Input: dimensioned drawing with shaded views. Units: mm. Origin: part minimum x, y, z. A direction names the side the tool comes from. Round coordinates to 2 decimals unless told otherwise and drop trailing zeros. Write each loop counter-clockwise with the first axis right and the second up, starting at its lowest first coordinate (ties: lowest second). Pieces come first, ordered by that corner, then holes. Notation, with made-up numbers: M 81,-35 L 136,-35 A22 cw 136,-3 Z; hole C 53,83 d7. An arc over 180 degrees is marked long. Put each result on its own line as item: value. Start each with the question number.
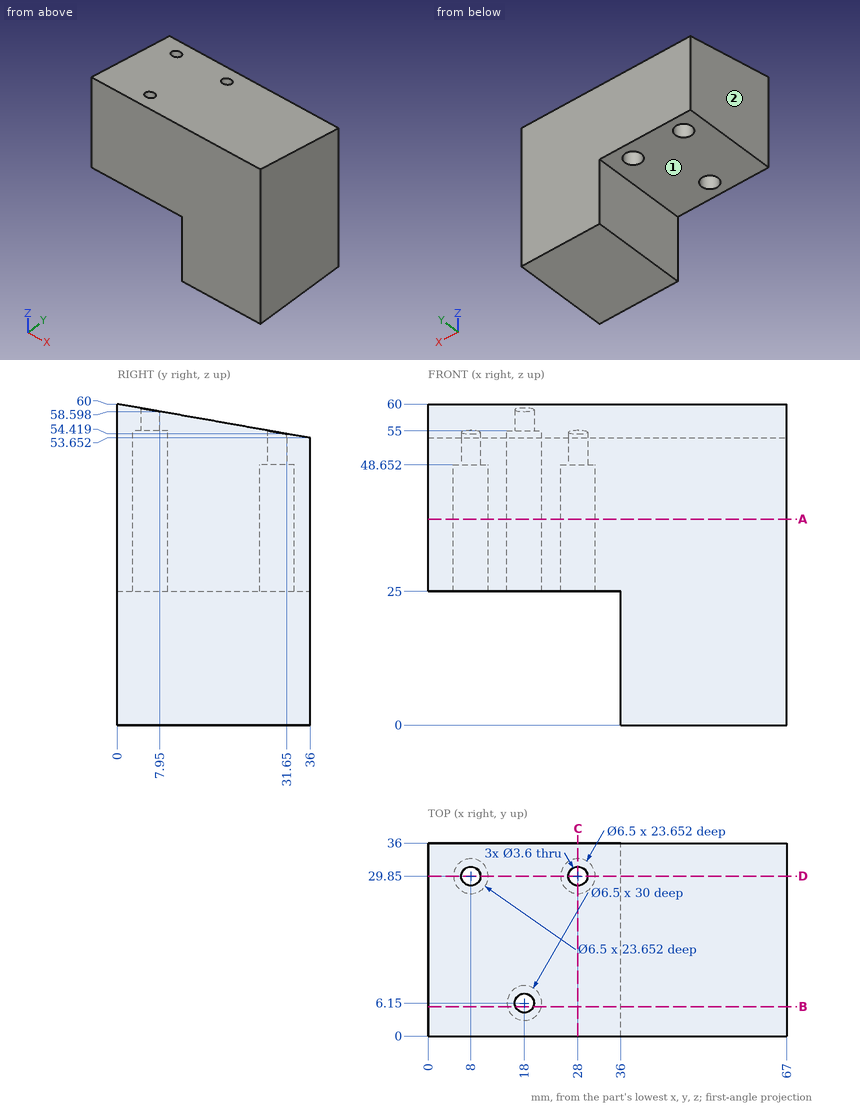
1) Access query for the marked faces 1 and 2. Directions: +Z, -Z, +X, -X, +Y, -Y. A direction counts if a zero-diameter tool reaches every point of the face in a straight line with its end or side. Return the directions, or none.
2) Section C-C, the plane x = 28. Output: boundary loops of the cut face in (y, z).
3) Ray query, probe 1 along X at (y, z) = (29.85, 51.5); probe 2 along X at (y, z) = (29, 35); probe 3 along Y at (x, z) = (18, 31). Return the intervals inside material, ascending.
4) Section A-A, the plane z = 38.5. Output: boundary loops of the cut face in (x, y), and give its area (3 significant figures).
5) First-contact query: pin 1 (7.5 mm diameter, centred on x = 8, y = 29.85, fed in from -Z); pin 2 (6 mm diameter, centred on x = 18, y = 6.15, fed in from +Z); pin 3 (4.5 mm diameter, centred on x = 8, y = 29.85, fed in from -Z); pin 4 (2 mm diameter, centred on x = 8, y = 30.5, fed in from -Z). Flat tips, straight axial feed; report the tip coordinate or a pass-through.
6) Section B-B, the plane y = 5.5. Output: boundary loops of the cut face in (x, z), and give its area (3 significant figures).
7) Section D-D, the plane y = 29.85. Output: boundary loops of the cut face in (x, z), and give its area (3 significant figures).
Solved:
1. face 1: -Z, -X, +Y, -Y
1. face 2: +Z, -Z, -X, +Y, -Y
2. outline: M 0,25 L 26.6,25 L 26.6,48.65 L 28.05,48.65 L 28.05,55.05 L 0,60 Z; M 31.65,48.65 L 33.1,48.65 L 33.1,25 L 36,25 L 36,53.65 L 31.65,54.42 Z
3. probe 1: x = 0 to 6.2, 9.8 to 26.2, 29.8 to 67
3. probe 2: x = 0 to 4.86, 11.14 to 24.86, 31.14 to 67
3. probe 3: y = 0 to 2.9, 9.4 to 36
4. outline: M 0,0 L 67,0 L 67,36 L 0,36 Z; hole C 8,29.85 d6.5; hole C 18,6.15 d6.5; hole C 28,29.85 d6.5
4. area: 2,310 mm2
5. pin 1: stops at z = 25
5. pin 2: stops at z = 59.44
5. pin 3: stops at z = 48.65
5. pin 4: passes through
6. outline: M 0,25 L 14.82,25 L 14.82,55 L 16.32,55 L 16.32,59.03 L 0,59.03 Z; M 19.68,55 L 21.18,55 L 21.18,25 L 36,25 L 36,0 L 67,0 L 67,59.03 L 19.68,59.03 Z
6. area: 2,850 mm2
7. outline: M 0,25 L 4.75,25 L 4.75,48.65 L 6.2,48.65 L 6.2,54.74 L 0,54.74 Z; M 9.8,48.65 L 11.25,48.65 L 11.25,25 L 24.75,25 L 24.75,48.65 L 26.2,48.65 L 26.2,54.74 L 9.8,54.74 Z; M 29.8,48.65 L 31.25,48.65 L 31.25,25 L 36,25 L 36,0 L 67,0 L 67,54.74 L 29.8,54.74 Z
7. area: 2,420 mm2
